Could you check a few things on this model? Use its own coordinates, in mm. Face numbers are marked on the shaded views. A direction names the side the tool comes from. Give positions to 0.01 mm unless a question says otherwise; leave off trailing zeros. Order: outer loops, then holes, each group sorted by start corner. A loop starts at its lowest first (then second) coordinate and runs counter-clockwise, first axis right, second up. Notation, with made-up numbers: M -13.5,-4.5 L 45.5,-4.5 A20 ccw 45.5,21.5 Z; hole C -24.75,-31.75 d2. An arc over 180 degrees is marked long. Use a Markdown table: item, result. Add a question column.
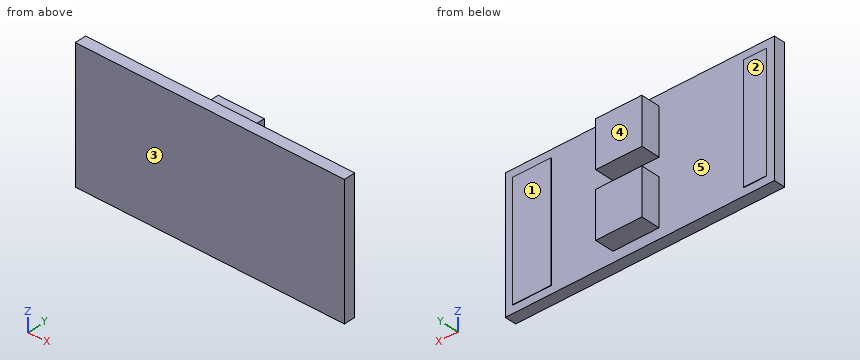
```python
from build123d import *

# Parameters (mm, degrees)
SKETCH_1_W      = 35
SKETCH_1_H      = 17
EXTRUDE_1_DEPTH = 1.5
SKETCH_4_W      = 6
SKETCH_4_H      = 6
EXTRUDE_3_DEPTH = 4
SKETCH_6_W      = 5
SKETCH_6_H      = 15
SKETCH_6_W_2    = 3
EXTRUDE_4_DEPTH = 1.55


with BuildPart() as part:
    # Эскиз1 → Бобышка-Вытянуть1 (new body)
    with BuildSketch(Plane(origin=(0, 0, 0), x_dir=(1, 0, 0), z_dir=(0, 1, 0))):
        with Locations((-17.5, 0)):
            Rectangle(SKETCH_1_W, SKETCH_1_H)
    extrude(amount=EXTRUDE_1_DEPTH)

    # Эскиз4 → Бобышка-Вытянуть3 (add)
    with BuildSketch(Plane(origin=(0, 0, 0), x_dir=(1, 0, 0), z_dir=(0, 1, 0))):
        with Locations((-17, 4.156615609)):
            Rectangle(SKETCH_4_W, SKETCH_4_H)
        with Locations((-17, -4.156615609)):
            Rectangle(SKETCH_4_W, SKETCH_4_H)
    extrude(amount=EXTRUDE_3_DEPTH)

    # Эскиз6 → Бобышка-Вытянуть4 (add)
    with BuildSketch(Plane(origin=(0, 0, 0), x_dir=(1, 0, 0), z_dir=(0, 1, 0))):
        with Locations((-3.5, 0)):
            Rectangle(SKETCH_6_W, SKETCH_6_H)
        with Locations((-32.5, 0)):
            Rectangle(SKETCH_6_W_2, SKETCH_6_H)
    extrude(amount=EXTRUDE_4_DEPTH)


solid = part.part
```
1) Suppose I cut it at C-C on z = -0.5. Please give me the cut outline in (x, y).
2) For the marked faces 1, 2 and 3, which set-ups out of +Z, -Z, +X, -X, +Y, -Y let a thin tool reach every point of the face, with its end or its side?
3) Suppose I cut it at A-A on y = 3.25. Please give me the cut outline in (x, z).
4) Please list where these lines run through material, in increasing order: line 1 (Y direction, x = -1.5, z = 4.5); line 2 (X direction, y = 2.4, z = -3.25); line 3 (Y direction, x = -23.5, z = -6). Write a range as from..to.
5) Suppose I cut it at D-D on x = -17.5. Please give me the cut outline in (y, z).
6) Suppose I cut it at B-B on x = -31.5. Please give me the cut outline in (y, z).
7) We'd pull the mould along X, two halves only. Please class the marked faces 4 and 5: pulls with the +X half, pulls with the -X half, needs draft (parallel to the pull), parting line crosses it, or undercut.
8) For pin 1 (2.5 mm diameter, centred on x = -3.5, z = -1.5, fed in from +Y); pin 2 (1.2 mm diameter, centred on y = 2.5, z = 5.5, fed in from +X); pin 3 (0.8 mm diameter, centred on x = -16, y = 3.5, fed in from +Z), each with a flat end and sliding along its axis, tell me the tip position at first contact or that it passes through.
Values found:
| question | item | result |
|---|---|---|
| 1 | outline | M -35,0 L 0,0 L 0,1.5 L -1,1.5 L -1,1.55 L -6,1.55 L -6,1.5 L -31,1.5 L -31,1.55 L -34,1.55 L -34,1.5 L -35,1.5 Z |
| 2 | face 1 | +Z, -Z, +X, +Y |
| 2 | face 2 | +Z, -Z, -X, +Y |
| 2 | face 3 | +Z, -Z, +X, -X, -Y |
| 3 | outline | M -20,-7.16 L -14,-7.16 L -14,-1.16 L -20,-1.16 Z; M -20,1.16 L -14,1.16 L -14,7.16 L -20,7.16 Z |
| 4 | line 1 | y = 0..1.55 |
| 4 | line 2 | x = -20..-14 |
| 4 | line 3 | y = 0..1.5 |
| 5 | outline | M 0,-8.5 L 1.5,-8.5 L 1.5,-7.16 L 4,-7.16 L 4,-1.16 L 1.5,-1.16 L 1.5,1.16 L 4,1.16 L 4,7.16 L 1.5,7.16 L 1.5,8.5 L 0,8.5 Z |
| 6 | outline | M 0,-8.5 L 1.5,-8.5 L 1.5,-7.5 L 1.55,-7.5 L 1.55,7.5 L 1.5,7.5 L 1.5,8.5 L 0,8.5 Z |
| 7 | face 4 | needs draft |
| 7 | face 5 | undercut |
| 8 | pin 1 | stops at y = 1.55 |
| 8 | pin 2 | stops at x = -14 |
| 8 | pin 3 | stops at z = 7.16 |
